```python
from build123d import *

# Parameters (mm, degrees)
F0_W           = 97.2000025213
F0_H           = 56.100005284
F1_DEPTH       = 25
F5_D           = 11
F5_CBORE_D     = 17.25
F5_CBORE_DEPTH = 10
F6_D           = 8.8
F6_START       = 7.1981119
F6_CBORE_D     = 14.25
F6_CBORE_DEPTH = 8


with BuildPart() as f1:
    # F0 (on Front) → F1 (new body)
    with BuildSketch(Plane.XZ):
        with Locations((-4.0499996394, 4.0500005707)):
            Rectangle(F0_W, F0_H)
    extrude(amount=F1_DEPTH)

    # F5 (through all)
    with Locations(Plane(origin=(0, 0, 0), x_dir=(-1, 0, 0), z_dir=(0, 1, 0))):
        with Locations((-30.8541376144, 17.6449194551)):
            CounterBoreHole(F5_D / 2, F5_CBORE_D / 2, F5_CBORE_DEPTH)

    # F6 (through all)
    # its depths count from where the whole tool has entered the part; down to there all is cleared
    with Locations(Plane(origin=(-42.3750020564, 0, 42.3750020564), x_dir=(0, 1, 0), z_dir=(-0.7071067812, 0, 0.7071067812)).offset(-F6_START)):
        with Locations((-12.6984147355, 14.4579308107)):
            CounterBoreHole(F6_D / 2, F6_CBORE_D / 2, F6_CBORE_DEPTH)


solid = f1.part
```
The listing builds one solid part. Answer for the finished solid, in the listing's coordinates (mm). A direction names the side the tool comes from. Give positions to 0.01 mm unless a question says otherwise; leave off trailing zeros. Loops run counter-clockwise (first coordinate to the right, second up) from the corner with the lowest first, then second, coordinate; pieces in that order, holes last. Notation, with made-up numbers: M 65,52.25 L 123,52.25 A29 cw 123,84.25 Z; hole C 35.5,10.5 d11. An arc over 180 degrees is marked long. One line per item, written item: value.
Q1. A cutting plane is placed at B-B on y = -22.75. Determine the outline of the cut face in (x, z).
Working result:
outline: M -52.65,-24 L 44.55,-24 L 44.55,32.1 L -52.65,32.1 Z; hole C 30.85,17.64 d11
Q2. A cutting plane is placed at D-D on y = -3.5. Determine the outline of the cut face in (x, z) (3 decimals).
Working result:
outline: M -52.65,-24 L 44.55,-24 L 44.55,32.1 L -52.65,32.1 Z; hole C 30.854,17.645 d17.25
Q3. For faces 1 (the face through (22.63, -4.93, 20.24)), 2 (the face through (-5, -12, 32.1)), determine the directions among +Z, -Z, +X, -X, +Y, -Y from which every point of the face is accessible in a straight line to the end or side of a thin tool.
Working result:
face 1: +Y
face 2: +Z, +X, -X, +Y, -Y
Q4. Find the intervals of material crossed by line 1 (X direction, y = -14.5, z = 15); line 2 (Z direction, x = -29, y = -11.5); line 3 (X direction, y = -15.75, z = 22), in increasing order. Write a range as from..to.
Working result:
line 1: x = -52.65..-41.12, -29.77..26.03, 35.68..44.55
line 2: z = -24..2.57, 14.54..32.1
line 3: x = -52.65..-51.55, -37.96..27.5, 34.21..44.55
Q5. A cutting plane is placed at C-C on y = -18.25. Determine the outline of the cut face in (x, z), then the cut area to 3 significant figures.
Working result:
outline: M -52.65,-24 L 44.55,-24 L 44.55,32.1 L -46.23,32.1 L -38.69,24.56 L -45.01,18.25 L -52.65,25.89 Z; hole C 30.85,17.64 d11
area: 5,240 mm^2
Q6. A cutting plane is placed at A-A on x = 28. Determine the outline of the cut face in (y, z), then the cut area to 3 significant figures.
Working result:
outline: M -25,-24 L 0,-24 L 0,9.51 L -10,9.51 L -10,12.94 L -25,12.94 Z; M -25,22.35 L -10,22.35 L -10,25.78 L 0,25.78 L 0,32.1 L -25,32.1 Z
area: 1,100 mm^2
Q7. Determine the mould class of faces 3 (the face through (-41.922, -8.048, 21.334)), 4 (the face through (-5, 0, 4)), 5 (the face through (-5, -12, -24)) for opening direction Y: +Y half, -Y half, draft (parallel to the pull), parting line (faces both ways), or undercut.
Working result:
face 3: undercut
face 4: +Y half
face 5: draft
